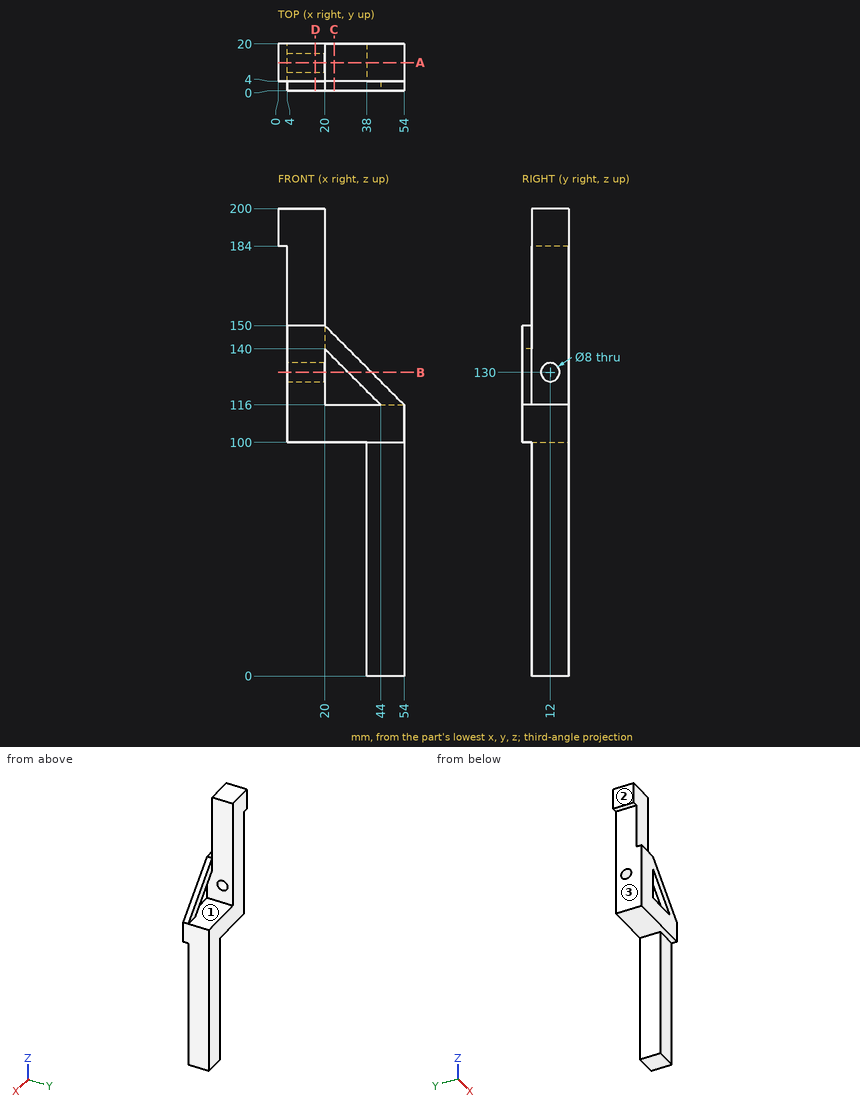
The figure shows three views and two pictorial views of one solid part (mm, origin at its lowest corner). Answer the questions. A direction names the side the tool comes from. Give positions to 0.01 mm unless a question says otherwise; leave off trailing zeros. Write each loop counter-clockwise with the first axis right and the second up, starting at its lowest first coordinate (ties: lowest second). Pieces come first, ordered by that corner, then holes. Notation, with made-up numbers: (-32.75, -10) -> (-24.75, -10) arc R16 cw to (-24.75, -2) -> close; hole circle Ø4 at (-35, -38.75). An arc over 180 degrees is marked (long way). Answer as a JSON object with one key per item and string values.
1) Section C-C on x = 24 is taken. Write down the section's boundary in (y, z), then the cut area to 3 significant figures.
Findings below:
{"outline": "(0, 100) -> (20, 100) -> (20, 116) -> (0, 116) -> close; (0, 136) -> (4, 136) -> (4, 146) -> (0, 146) -> close", "area": "360 mm^2"}
2) Section B-B on z = 130 is taken. Write down the section's boundary in (x, y).
Findings below:
{"outline": "(4, 0) -> (20, 0) -> (20, 8) -> (4, 8) -> close; (4, 16) -> (20, 16) -> (20, 20) -> (4, 20) -> close; (30, 0) -> (40, 0) -> (40, 4) -> (30, 4) -> close"}
3) A tool of negligible diameter and unlimited length cuts with its end or side. For the marked faces 1, 2 and 3, from which of +Z, -Z, +X, -X, +Y, -Y can it reach the whole face along a straight path? Write none if from no direction.
Findings below:
{"face 1": "+Y", "face 2": "+Z, -Z, -X, +Y, -Y", "face 3": "-Z, -X, +Y, -Y"}
4) Section A-A on y = 12 is taken. Write down the section's boundary in (x, z), then the cut area to 3 significant figures.
Findings below:
{"outline": "(0, 184) -> (4, 184) -> (4, 134) -> (20, 134) -> (20, 200) -> (0, 200) -> close; (4, 100) -> (38, 100) -> (38, 0) -> (54, 0) -> (54, 116) -> (20, 116) -> (20, 126) -> (4, 126) -> close", "area": "3,680 mm^2"}
5) Section D-D on x = 16 is taken. Write down the section's boundary in (y, z).
Findings below:
{"outline": "(0, 100) -> (20, 100) -> (20, 200) -> (4, 200) -> (4, 150) -> (0, 150) -> close; hole circle Ø8 at (12, 130)"}
6) Flat-ended cylindrical pins translate along their axes: pin 1 Ø5 at (x, y) = (11.5, 4.5) entering from -Z; pin 2 Ø10 at (y, z) = (8.5, 153) entering from -X; pin 3 Ø5 at (x, z) = (43, 52.5) entering from -Y. Find the tip coordinate at first contact, or state that the pin passes through.
Findings below:
{"pin 1": "stops at z = 100", "pin 2": "stops at x = 4", "pin 3": "stops at y = 4"}
7) Straight lines are drawn through the part: probe 1 along Y at (x, z) = (15.5, 130); probe 2 along Z at (x, y) = (14.75, 12); probe 3 along Y at (x, z) = (15, 169). For each, find the intervals that lie inside material, in ascending order. Write a range as from..to.
Findings below:
{"probe 1": "y = 0..8, 16..20", "probe 2": "z = 100..126, 134..200", "probe 3": "y = 4..20"}
